For this review, take the finished solid that the model builds, in its own axes (mm). Face numbers are marked on the shaded views. Round coordinates to 2 decimals unless told otherwise and drop trailing zeros. Write each loop counter-clockwise with the first axis right and the second up, starting at its lowest first coordinate (ties: lowest second). Pieces come first, ordered by that corner, then holes.
from build123d import *

# Parameters (mm, degrees)
BRIDA_D3_25IN_1_4IN_START          = 413.9
CROQUIS1_R                         = 41.275
BRIDA_D3_25IN_1_4IN_DEPTH          = 6.35
BARRENOS_SALIDA_M6_START           = 413.9
CROQUIS2_R                         = 1.45
CROQUIS2_R_2                       = 5
BARRENOS_SALIDA_M6_DEPTH           = 6.35
REFRENTADO_M2_5_START              = 417.65
CROQUIS3_R                         = 2.5
REFRENTADO_M2_5_DEPTH              = 2.6
ISO9409_50_4XM6_Y_PASADOR_D6_START = 413.9
CROQUIS4_R                         = 2.5
CROQUIS4_R_2                       = 3
ISO9409_50_4XM6_Y_PASADOR_D6_DEPTH = 6.35
PATRON_8XM4_PCD2_5IN_START         = 413.9
CROQUIS5_R                         = 1.65
PATRON_8XM4_PCD2_5IN_DEPTH         = 6.35
PATRON_6XM3_PCD40_START            = 413.9
CROQUIS6_R                         = 1.25
PATRON_6XM3_PCD40_DEPTH            = 6.35


with BuildPart() as part:
    # Croquis1 → Brida_D3-25in_1-4in (new body)
    with BuildSketch(Plane.XY.offset(BRIDA_D3_25IN_1_4IN_START)):
        with Locations((152.4, 0)):
            Circle(CROQUIS1_R)
    extrude(amount=BRIDA_D3_25IN_1_4IN_DEPTH)

    # Croquis2 → Barrenos_salida_M6 (cut)
    with BuildSketch(Plane.XY.offset(BARRENOS_SALIDA_M6_START)):
        with Locations((159.426042223, 10.338507178)):
            Circle(CROQUIS2_R)
        with Locations((146.959611258, 11.253984643)):
            Circle(CROQUIS2_R)
        with Locations((139.933569035, 0.915477464)):
            Circle(CROQUIS2_R)
        with Locations((145.373957777, -10.338507178)):
            Circle(CROQUIS2_R)
        with Locations((157.840388742, -11.253984643)):
            Circle(CROQUIS2_R)
        with Locations((164.866430965, -0.915477464)):
            Circle(CROQUIS2_R)
        with Locations((152.4, 0)):
            Circle(CROQUIS2_R_2)
    extrude(amount=BARRENOS_SALIDA_M6_DEPTH, mode=Mode.SUBTRACT)

    # Croquis3 → Refrentado_M2-5 (cut)
    with BuildSketch(Plane.XY.offset(REFRENTADO_M2_5_START)):
        with Locations((159.426042223, 10.338507178)):
            Circle(CROQUIS3_R)
        with Locations((146.959611258, 11.253984643)):
            Circle(CROQUIS3_R)
        with Locations((139.933569035, 0.915477464)):
            Circle(CROQUIS3_R)
        with Locations((145.373957777, -10.338507178)):
            Circle(CROQUIS3_R)
        with Locations((157.840388742, -11.253984643)):
            Circle(CROQUIS3_R)
        with Locations((164.866430965, -0.915477464)):
            Circle(CROQUIS3_R)
    extrude(amount=REFRENTADO_M2_5_DEPTH, mode=Mode.SUBTRACT)

    # Croquis4 → ISO9409-50_4xM6_y_pasador_D6 (cut)
    with BuildSketch(Plane.XY.offset(ISO9409_50_4XM6_Y_PASADOR_D6_START)):
        with Locations((170.07766953, 17.67766953)):
            Circle(CROQUIS4_R)
        with Locations((134.72233047, 17.67766953)):
            Circle(CROQUIS4_R)
        with Locations((134.72233047, -17.67766953)):
            Circle(CROQUIS4_R)
        with Locations((170.07766953, -17.67766953)):
            Circle(CROQUIS4_R)
        with Locations((152.4, 25)):
            Circle(CROQUIS4_R_2)
    extrude(amount=ISO9409_50_4XM6_Y_PASADOR_D6_DEPTH, mode=Mode.SUBTRACT)

    # Croquis5 → Patron_8xM4_PCD2-5in (cut)
    with BuildSketch(Plane.XY.offset(PATRON_8XM4_PCD2_5IN_START)):
        with Locations((181.733175157, 12.150198978)):
            Circle(CROQUIS5_R)
        with Locations((164.550198978, 29.333175157)):
            Circle(CROQUIS5_R)
        with Locations((140.249801022, 29.333175157)):
            Circle(CROQUIS5_R)
        with Locations((123.066824843, 12.150198978)):
            Circle(CROQUIS5_R)
        with Locations((123.066824843, -12.150198978)):
            Circle(CROQUIS5_R)
        with Locations((140.249801022, -29.333175157)):
            Circle(CROQUIS5_R)
        with Locations((164.550198978, -29.333175157)):
            Circle(CROQUIS5_R)
        with Locations((181.733175157, -12.150198978)):
            Circle(CROQUIS5_R)
    extrude(amount=PATRON_8XM4_PCD2_5IN_DEPTH, mode=Mode.SUBTRACT)

    # Croquis6 → Patron_6xM3_PCD40 (cut)
    with BuildSketch(Plane.XY.offset(PATRON_6XM3_PCD40_START)):
        with Locations((172.4, 0)):
            Circle(CROQUIS6_R)
        with Locations((162.4, 17.320508076)):
            Circle(CROQUIS6_R)
        with Locations((142.4, 17.320508076)):
            Circle(CROQUIS6_R)
        with Locations((132.4, 0)):
            Circle(CROQUIS6_R)
        with Locations((142.4, -17.320508076)):
            Circle(CROQUIS6_R)
        with Locations((162.4, -17.320508076)):
            Circle(CROQUIS6_R)
    extrude(amount=PATRON_6XM3_PCD40_DEPTH, mode=Mode.SUBTRACT)


solid = part.part
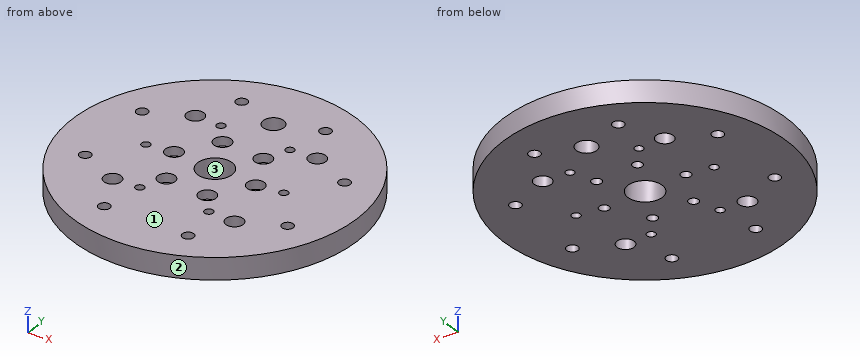
(1) We need section A-A, the plane x = 152.4. Give the boundary of the cut face in (y, z) (3 decimals), and give its area (3 significant figures).
Geometry check:
outline: (-41.275, 413.9) - (-5, 413.9) - (-5, 420.25) - (-41.275, 420.25) - close; (5, 413.9) - (22, 413.9) - (22, 420.25) - (5, 420.25) - close; (28, 413.9) - (41.275, 413.9) - (41.275, 420.25) - (28, 420.25) - close
area: 423 mm2
(2) We need section D-D, the plane y = -36. Give the boundary of the cut face in (x, z), and give its area (3 significant figures).
Geometry check:
outline: (132.21, 413.9) - (172.59, 413.9) - (172.59, 420.25) - (132.21, 420.25) - close
area: 256 mm2
(3) For line 1 along Y through (x, z) = (141, 416.75); line 2 along Y through (x, z) = (166, 414.5); line 3 along X through (y, z) = (17, 418.75), list the stretches that pass through material, from the lowest coordinate up.
Geometry check:
line 1: y = -39.67 to -30.8, -27.86 to -0.07, 1.9 to 27.86, 30.8 to 39.67
line 2: y = -38.97 to -30.12, -28.55 to -1.82, -0.01 to 28.55, 30.12 to 38.97
line 3: x = 114.79 to 132.32, 137.13 to 141.19, 143.61 to 161.19, 163.61 to 167.67, 172.48 to 190.01
(4) For pin 1 Ø1.5 at (x, y) = (139.5, 1) entering from +Z; pin 2 Ø4.5 at (x, y) = (123.07, -12.15) entering from -Z; pin 3 Ø1.5 at (x, z) = (168.5, 417) entering from -Y; pin 4 Ø3 at (x, z) = (119.5, 414.5) entering from +Y, all flat-tipped, find the tip position at first contact; note any pin that passes through.
Geometry check:
pin 1: passes through
pin 2: stops at z = 413.9
pin 3: stops at y = -38.31
pin 4: stops at y = 26.79
(5) We need section B-B, the plane y = 25. Give the boundary of the cut face in (x, z).
Geometry check:
outline: (119.56, 413.9) - (149.4, 413.9) - (149.4, 420.25) - (119.56, 420.25) - close; (155.4, 413.9) - (185.24, 413.9) - (185.24, 420.25) - (155.4, 420.25) - close
(6) Mouldability with a two-part tool opening along X and no side actions: class the marked faces 1, 2 and 3 as pulls with the +X half, pulls with the -X half, needs draft (parallel to the pull), parting line crosses it, or undercut.
Geometry check:
face 1: needs draft
face 2: parting line crosses it
face 3: undercut
(7) We need section C-C, the plane x = 184.5. Give the boundary of the cut face in (y, z).
Geometry check:
outline: (-25.95, 413.9) - (25.95, 413.9) - (25.95, 420.25) - (-25.95, 420.25) - close
